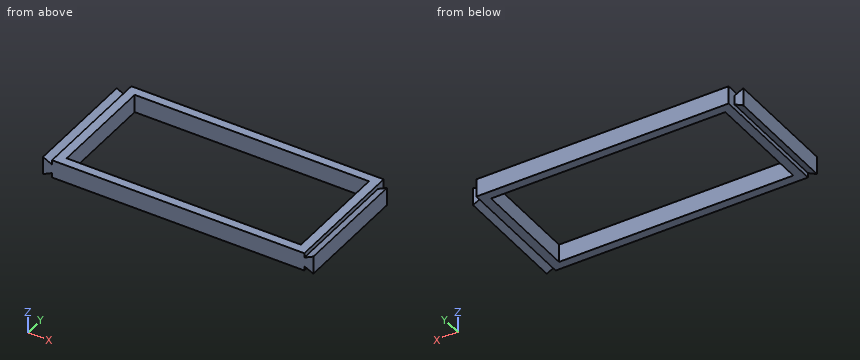
Autodesk Inventor part; units mm, degrees
ref_plane "YZ Plane" through (0, 0, 0) normal (1, 0, 0) x (0, 1, 0)
ref_plane "XZ Plane" through (0, 0, 0) normal (0, 1, 0) x (-1, 0, 0)
ref_plane "XY Plane" through (0, 0, 0) normal (0, 0, 1) x (1, 0, 0)
sketch "Sketch1" plane through (0, 0, 0) normal (0, 1, 0) x (-1, 0, 0)
  line L0 (0, 0) -> (-177.8, 0)
  line L1 (-177.8, 0) -> (-177.8, -12.7)
  line L2 (-177.8, -12.7) -> (0, -12.7)
  line L3 (0, -12.7) -> (0, 0)
  dimension "d0" = 177.8
  dimension "d1" = 12.7
extrude "Extrusion1" add sketch "Sketch1" along normal blind 88.9
sketch "Sketch2" plane through (0, 0, 0) normal (0, 1, 0) x (-1, 0, 0)
  line L0 (0, -12.7) -> (0, 0) construction
  line L1 (0, -12.6308) -> (0, 0) construction
  line L2 (0, -6.3154) -> (6.35, -6.3154) construction
  line L3 (6.35, 0) -> (6.35, -12.6308)
  line L4 (0, -6.3154) -> (0, -3.1658)
  line L5 (0, -6.3154) -> (0, -9.465)
  line L6 (0, -9.465) -> (6.35, -12.6308)
  line L7 (0, -3.1658) -> (6.35, 0)
  line L8 (-177.8, -12.7) -> (0, -12.7) construction
  line L9 (-88.9, -12.7) -> (-88.9, 0) construction
  line L10 (-177.8, -12.7) -> (-177.8, 0) construction
  line L11 (-184.15, 0) -> (-184.15, -12.6308)
  line L12 (-177.8, -9.465) -> (-184.15, -12.6308)
  line L13 (-177.8, -3.1658) -> (-184.15, 0)
  line L14 (-177.8, -9.465) -> (-177.8, -3.1658)
  line L15 (0, -9.465) -> (0, -3.1658)
  line L16 (-177.8, -9.465) -> (-184.15, -12.6308)
  line L17 (-184.15, 0) -> (-177.8, -3.1658)
  dimension "d4" = 6.35
  dimension "d5" = 3.1496
  dimension "d6" = 3.1496
  dimension "d9" = 12.6308
extrude "Extrusion2" add sketch "Sketch2" along normal blind 82.55
sketch "Sketch3" plane through (0, 0, 0) normal (0, 0, 1) x (1, 0, 0)
  line L0 (0, 0) -> (177.8, 0)
  line L1 (177.8, 0) -> (177.8, 88.9)
  line L2 (0, 88.9) -> (177.8, 88.9)
  line L3 (0, 0) -> (0, 88.9)
  line L4 (171.45, 82.55) -> (171.45, 6.35)
  line L5 (171.45, 6.35) -> (6.35, 6.35)
  line L6 (31.75, 82.55) -> (31.75, 6.35)
  line L7 (6.35, 6.35) -> (6.35, 82.55)
  line L8 (6.35, 82.55) -> (171.45, 82.55)
  line L9 (38.1, 82.55) -> (38.1, 6.35)
  line L10 (63.5, 82.55) -> (63.5, 6.35)
  line L11 (69.85, 82.55) -> (69.85, 6.35)
  line L12 (95.25, 82.55) -> (95.25, 6.35)
  line L13 (101.6, 82.55) -> (101.6, 6.35)
  line L14 (127, 82.55) -> (127, 6.35)
  line L15 (133.35, 82.55) -> (133.35, 6.35)
  line L16 (158.75, 82.55) -> (158.75, 6.35)
  line L17 (165.1, 82.55) -> (165.1, 6.35)
  line L18 (6.35, 82.55) -> (171.45, 82.55)
  line L19 (171.45, 82.55) -> (171.45, 6.35)
  line L20 (171.45, 6.35) -> (6.35, 6.35)
  line L21 (6.35, 6.35) -> (6.35, 82.55)
  dimension "d12" = 6.35
  dimension "d13" = 25.4
  dimension "d14" = 6.35
  dimension "d15" = 25.4
  dimension "d16" = 6.35
  dimension "d17" = 25.4
  dimension "d18" = 6.35
  dimension "d19" = 25.4
  dimension "d20" = 6.35
extrude "Extrusion3" cut sketch "Sketch3" against normal blind 76.2 contours L4 L5 L17 L8 | L17 L5 L16 L8 | L16 L5 L15 L8 | L15 L5 L14 L8 | L14 L5 L13 L8 | L13 L5 L12 L8 | L12 L5 L11 L8 | L11 L5 L10 L8 | L10 L5 L9 L8 | L9 L5 L6 L8 | L6 L5 L7 L8
properties part number "doveTailBar"
For this review, take the finished solid that the model builds, in its own axes (mm). Coordinates: 2 decimals unless noted, no trailing zeros. Order: outer loops, then holes, each group sorted by start corner. A loop starts at its lowest first (then second) coordinate and runs counter-clockwise, first axis right, second up. Notation, with made-up numbers: (42.5, -17.5) - (100.5, -17.5) arc R14 ccw to (100.5, -12.5) - close; hole circle Ø6 at (-16, 73.25). An arc over 180 degrees is marked (long way). Answer as CSV lines item,"result". Start each with the question number.
1) Add section A-A (y = 37.5). State the section outline as (x, z) points (3 decimals).
2) Insertion check: P1, Ø5, axis at x = 37, z = -2, coming from the -Y side; P2, Ø1.9, axis at x = 182, z = -5.5, coming from the +Y side. Each pin has a flat end and moves straight along its axis. Give the tip position at first contact, or say it passes through.
3) To check wall thickness, follow line 1 along Y through (x, z) = (155, -11.25); line 2 along X through (y, z) = (27, -6); line 3 along X through (y, z) = (38, -11.5). State the ranges of each line that lie inside material, in increasing order. Write a range as [from, to].
4) Add section B-B (x = 63.5). State the section outline as (y, z) points, then the cut area to 3 significant figures.
5) Add section C-C (z = -6.75). State the section outline as (x, y) points.
Result:
1,outline,"(-6.35, -12.631) - (0, -9.465) - (0, -12.7) - (6.35, -12.7) - (6.35, 0) - (0, 0) - (0, -3.166) - (-6.35, 0) - close; (171.45, -12.7) - (177.8, -12.7) - (177.8, -9.465) - (184.15, -12.631) - (184.15, 0) - (177.8, -3.166) - (177.8, 0) - (171.45, 0) - close"
2,P1,"y = 0"
2,P2,"y = 82.55"
3,line 1,"[0, 6.35], [82.55, 88.9]"
3,line 2,"[-6.35, 6.35], [171.45, 184.15]"
3,line 3,"[-6.35, -4.08], [0, 6.35], [171.45, 177.8], [181.88, 184.15]"
4,outline,"(0, -12.7) - (6.35, -12.7) - (6.35, 0) - (0, 0) - close; (82.55, -12.7) - (88.9, -12.7) - (88.9, 0) - (82.55, 0) - close"
4,area,"161 mm^2"
5,outline,"(-6.35, 0) - (184.15, 0) - (184.15, 82.55) - (177.8, 82.55) - (177.8, 88.9) - (0, 88.9) - (0, 82.55) - (-6.35, 82.55) - close; hole (6.35, 6.35) - (171.45, 6.35) - (171.45, 82.55) - (6.35, 82.55) - close"
